CAD build for the part. Positions are in the model's coordinates, mm. A direction names the side the tool comes from. Round coordinates to 2 decimals unless told otherwise and drop trailing zeros. Loops run counter-clockwise (first coordinate to the right, second up) from the corner with the lowest first, then second, coordinate; pieces in that order, holes last. Notation, with made-up numbers: (-28, 31.5) -> (15, 31.5) arc R28 cw to (15, 50.5) -> close; hole circle Ø7 at (-30.75, 36). An arc over 180 degrees is marked (long way). Answer as CSV lines item,"result".
```python
from build123d import *

# Parameters (mm, degrees)
CROQUIS1_W              = 11
CROQUIS1_H              = 33
SALIENTE_EXTRUIR1_DEPTH = 33
CROQUIS2_W              = 11
CROQUIS2_H              = 17
CORTAR_EXTRUIR1_DEPTH   = 6
CORTAR_EXTRUIR2_REACH   = 13
SALIENTE_EXTRUIR4_DEPTH = 5
CROQUIS7_R              = 2.3
SALIENTE_EXTRUIR5_DEPTH = 3
CROQUIS8_R              = 1
CORTAR_EXTRUIR4_DEPTH   = 3
CROQUIS9_W              = 1
CROQUIS9_H              = 21
CORTAR_EXTRUIR5_DEPTH   = 20


with BuildPart() as part:
    # Croquis1 → Saliente-Extruir1 (new body)
    with BuildSketch(Plane.XY):
        Rectangle(CROQUIS1_W, CROQUIS1_H)
    extrude(amount=SALIENTE_EXTRUIR1_DEPTH)

    # Croquis2 → Cortar-Extruir1 (cut)
    with BuildSketch(Plane.XZ.offset(16.5)):
        with Locations((0, 8.5)):
            Rectangle(CROQUIS2_W, CROQUIS2_H)
    cortar_extruir1 = extrude(amount=-CORTAR_EXTRUIR1_DEPTH, mode=Mode.SUBTRACT)

    # Simetría1: Cortar-Extruir1 across plane
    add(cortar_extruir1.mirror(Plane.ZX), mode=Mode.SUBTRACT)

    # Croquis3 → Cortar-Extruir2 (cut, up to next)
    with BuildSketch(Plane(origin=(5.5, 0, 0), x_dir=(0, 0, -1), z_dir=(1, 0, 0)), mode=Mode.PRIVATE) as cortar_extruir2_sk1:
        Polygon((-19, -16.5), (-19, -10.530920557), (-23.005061079, -10.530920557), (-23.005061079, 10.5), (-19, 10.5), (-19, 16.5), (-33, 16.5), (-33, -16.5), align=None)
    cortar_extruir2_tool1 = extrude(cortar_extruir2_sk1.sketch, amount=-CORTAR_EXTRUIR2_REACH, mode=Mode.PRIVATE) & part.part
    add(cortar_extruir2_tool1.solids().sort_by_distance((5.5, 0.003447, 27.11427))[0], mode=Mode.SUBTRACT)

    # Croquis6 → Saliente-Extruir4 (add)
    with BuildSketch(Plane.XY.offset(23.005061079)):
        with BuildLine():
            Line((-1.964593249, 1.559922557), (-1.964593249, 0.194840348))
            ThreePointArc((-1.964593249, 0.194840348), (0, -10.442315807), (1.964593249, 0.194840348))
            Line((1.964593249, 0.194840348), (1.964593249, 1.559922557))
            ThreePointArc((1.964593249, 1.559922557), (0, 3.524515805), (-1.964593249, 1.559922557))
        make_face()
    extrude(amount=SALIENTE_EXTRUIR4_DEPTH)

    # Croquis7 → Saliente-Extruir5 (add)
    with BuildSketch(Plane.XY.offset(28.005061079)):
        with Locations((0.048442296, -8.079125274)):
            Circle(CROQUIS7_R)
    extrude(amount=SALIENTE_EXTRUIR5_DEPTH)

    # Croquis8 → Cortar-Extruir4 (cut)
    with BuildSketch(Plane.XY.offset(19)):
        with Locations((0, -13.530920557)):
            Circle(CROQUIS8_R)
        with Locations((0, 13.530920557)):
            Circle(CROQUIS8_R)
    extrude(amount=-CORTAR_EXTRUIR4_DEPTH, mode=Mode.SUBTRACT)

    # Croquis9 → Cortar-Extruir5 (cut)
    with BuildSketch(Plane(origin=(5.5, 0, 0), x_dir=(0, 0, -1), z_dir=(1, 0, 0))):
        with Locations((-0.5, 0)):
            Rectangle(CROQUIS9_W, CROQUIS9_H)
    extrude(amount=-CORTAR_EXTRUIR5_DEPTH, mode=Mode.SUBTRACT)


solid = part.part
```
Q1. Two-plate mould, pull along Y, no slides. Class faces 4 (the cylindrical face through (-0.21, -10.44, 25.47)), 5 (the flat face through (0, 10.5, 21)), 6 (the flat face through (1.3, -13.6, 19)), 7 (the cylindrical face through (-0.13, 14.522, 18.014)): pulls with the +Y half, pulls with the -Y half, needs draft (parallel to the pull), parting line crosses it, or undercut.
Results:
face 4,"parting line crosses it"
face 5,"pulls with the +Y half"
face 6,"needs draft"
face 7,"undercut"
Q2. Slice it at A-A, the plane x = 0. Give the cut face in (y, z), and give its area (3 significant figures).
Results:
outline,"(-16.5, 17) -> (-14.53, 17) -> (-14.53, 19) -> (-16.5, 19) -> close; (-12.53, 17) -> (-10.5, 17) -> (-10.5, 1) -> (10.5, 1) -> (10.5, 17) -> (12.53, 17) -> (12.53, 19) -> (10.5, 19) -> (10.5, 23.01) -> (3.52, 23.01) -> (3.52, 28.01) -> (-5.78, 28.01) -> (-5.78, 31.01) -> (-10.38, 31.01) -> (-10.38, 28.01) -> (-10.44, 28.01) -> (-10.44, 23.01) -> (-10.53, 23.01) -> (-10.53, 19) -> (-12.53, 19) -> close; (14.53, 17) -> (16.5, 17) -> (16.5, 19) -> (14.53, 19) -> close"
area,"562 mm2"
Q3. Slice it at B-B, the plane z = 25.5. Give the cut face in (x, y).
Results:
outline,"(-1.96, 0.19) arc R5.5 ccw (long way) to (1.96, 0.19) -> (1.96, 1.56) arc R1.96 ccw to (-1.96, 1.56) -> close"
Q4. Drop flat-ended pins along their axis: pin 1 Ø1.8 at (x, y) = (1, -14.5) entering from +Z; pin 2 Ø1.5 at (y, z) = (0.5, 25.5) entering from -X; pin 3 Ø4 at (x, z) = (0.5, 22) entering from -Y. Give the stop position or say it passes through.
Results:
pin 1,"z = 19"
pin 2,"x = -2.87"
pin 3,"y = -10.53"
Q5. Slice it at D-D, the plane y = 12. Give the cut face in (x, z), and give its area (3 significant figures).
Results:
outline,"(-5.5, 17) -> (5.5, 17) -> (5.5, 19) -> (-5.5, 19) -> close"
area,"22.0 mm2"
Q6. Slice it at C-C, the plane x = 4.75. Give the cut face in (y, z), and give its area (3 significant figures).
Results:
outline,"(-16.5, 17) -> (-10.5, 17) -> (-10.5, 1) -> (10.5, 1) -> (10.5, 17) -> (16.5, 17) -> (16.5, 19) -> (10.5, 19) -> (10.5, 23.01) -> (-2.17, 23.01) -> (-2.17, 28.01) -> (-7.71, 28.01) -> (-7.71, 23.01) -> (-10.53, 23.01) -> (-10.53, 19) -> (-16.5, 19) -> close"
area,"514 mm2"
Q7. Probe L1, parallel to Y at x = 0, z = 17.55; L2, parallel to Z at x = -2, y = 9; L3, parallel to Y at x = 4.25, z = 22.5. List the from-to ranges inside material, lowest first. Write a range as [from, to].
Results:
L1,"[-16.5, -14.53], [-12.53, 12.53], [14.53, 16.5]"
L2,"[1, 23.01]"
L3,"[-10.53, 10.5]"
Q8. Tool access for faces 1 (the flat face through (-1.3, 13.5, 17)), 2 (the flat face through (1.965, 1, 25)), 3 (the flat face through (1.3, 13.5, 19)): list every direction of +Z, -Z, +X, -X, +Y, -Y with a clear straight run to the whole face (end or side of a thin tool).
Results:
face 1,"-Z, +X, -X, +Y"
face 2,"+Z, +X, +Y"
face 3,"+Z, +X, -X, +Y"
